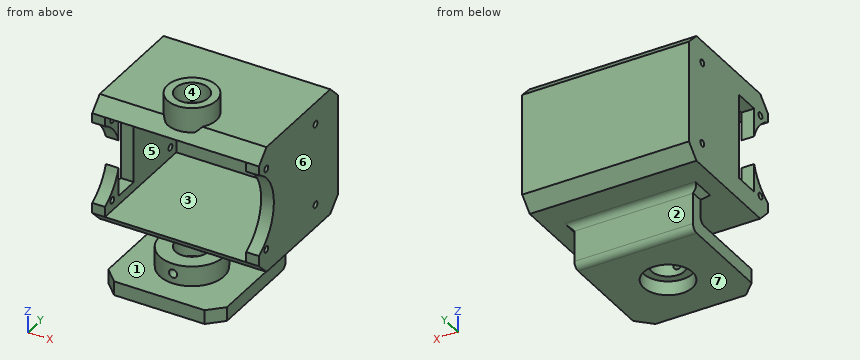
```python
from build123d import *

# Parameters (mm, degrees)
SKETCH1_W                       = 25
SKETCH1_H                       = 30
BOSS_EXTRUDE1_DEPTH             = 3.175
SKETCH2_W                       = 25
SKETCH2_H                       = 3.175
BOSS_EXTRUDE2_DEPTH             = 41.58
SKETCH3_W                       = 3.175
SKETCH3_H                       = 25
BOSS_EXTRUDE3_DEPTH             = 30
CUT_EXTRUDE1_REACH              = 60.775
SKETCH4_R                       = 11.5
CUT_EXTRUDE2_REACH              = 60.775
SKETCH5_R                       = 0.8
CUT_EXTRUDE3_REACH              = 60.775
SKETCH6_R                       = 0.8
SKETCH6_R_2                     = 0.799851166
SKETCH6_W                       = 21.2
SKETCH6_H                       = 6.375
CUT_EXTRUDE4_REACH              = 60.775
SKETCH7_R                       = 11.5
BOSS_EXTRUDE4_DEPTH             = 0.2
SKETCH9_W                       = 41.58
SKETCH9_H                       = 33.175
BOSS_EXTRUDE5_DEPTH             = 3.175
BOSS_EXTRUDE6_DEPTH             = 0.2
SKETCH11_W                      = 41.58
SKETCH11_H                      = 33.175
BOSS_EXTRUDE7_DEPTH             = 3.175
CHAMFER1_SIZE                   = 3.175
CHAMFER2_SIZE                   = 3.175
SKETCH13_W                      = 29.58
SKETCH13_H                      = 3.175
BOSS_EXTRUDE8_DEPTH             = 7.695
BOSS_EXTRUDE9_REACH             = 59.968
SKETCH14_W                      = 29.58
SKETCH14_H                      = 3.5
BOSS_EXTRUDE9_DIRECTION_2_DEPTH = 25
CHAMFER3_SIZE                   = 3.5
FILLET1_R                       = 1.5875
FILLET2_R                       = 1.5875
CUT_EXTRUDE5_REACH              = 70.161
SKETCH16_R                      = 6.1
SKETCH20_R                      = 8
SKETCH20_R_2                    = 4.1
BOSS_EXTRUDE11_DEPTH            = 5
CUT_EXTRUDE6_START              = -21.7275
SKETCH21_R                      = 1.025
CUT_EXTRUDE6_DEPTH              = 16
BOSS_EXTRUDE12_DEPTH            = 5
BOSS_EXTRUDE12_DEPTH_BACK       = 1.2
SKETCH23_R                      = 6.1
SKETCH23_R_2                    = 4.1
CHAMFER4_SIZE                   = 1.5


with BuildPart() as part:
    # Sketch1 → Boss-Extrude1 (new body)
    with BuildSketch(Plane(origin=(0, 0, 0), x_dir=(0, 0, -1), z_dir=(1, 0, 0))):
        with Locations((12.5, 15)):
            Rectangle(SKETCH1_W, SKETCH1_H)
    extrude(amount=BOSS_EXTRUDE1_DEPTH)

    # Sketch2 → Boss-Extrude2 (add)
    with BuildSketch(Plane.ZY):
        with Locations((-12.5, 31.5875)):
            Rectangle(SKETCH2_W, SKETCH2_H)
    extrude(amount=-BOSS_EXTRUDE2_DEPTH)

    # Sketch3 → Boss-Extrude3 (add)
    with BuildSketch(Plane.XZ.offset(-30)):
        with Locations((39.9925, -12.5)):
            Rectangle(SKETCH3_W, SKETCH3_H)
    extrude(amount=BOSS_EXTRUDE3_DEPTH)

    # Sketch4 → Cut-Extrude1 (cut, up to next)
    with BuildSketch(Plane.ZY, mode=Mode.PRIVATE) as cut_extrude1_sk1:
        with Locations((-12.359999929, -5.209996254)):
            Circle(SKETCH4_R)
    cut_extrude1_tool1 = extrude(cut_extrude1_sk1.sketch, amount=-CUT_EXTRUDE1_REACH, mode=Mode.PRIVATE) & part.part
    add(cut_extrude1_tool1.solids().sort_by_distance((0, -5.209996, -12.36))[0], mode=Mode.SUBTRACT)

    # Sketch5 → Cut-Extrude2 (cut, up to next)
    with BuildSketch(Plane.ZY, mode=Mode.PRIVATE) as cut_extrude2_sk1:
        with Locations((-22.609999929, 3.090003746)):
            Circle(SKETCH5_R)
    cut_extrude2_tool1 = extrude(cut_extrude2_sk1.sketch, amount=-CUT_EXTRUDE2_REACH, mode=Mode.PRIVATE) & part.part
    # Sketch5 → Cut-Extrude2 (cut, up to next)
    with BuildSketch(Plane.ZY, mode=Mode.PRIVATE) as cut_extrude2_sk2:
        with Locations((-22.609999929, 23.790003746)):
            Circle(SKETCH5_R)
    cut_extrude2_tool2 = extrude(cut_extrude2_sk2.sketch, amount=-CUT_EXTRUDE2_REACH, mode=Mode.PRIVATE) & part.part
    # Sketch5 → Cut-Extrude2 (cut, up to next)
    with BuildSketch(Plane.ZY, mode=Mode.PRIVATE) as cut_extrude2_sk3:
        with Locations((-2.109999929, 23.790003746)):
            Circle(SKETCH5_R)
    cut_extrude2_tool3 = extrude(cut_extrude2_sk3.sketch, amount=-CUT_EXTRUDE2_REACH, mode=Mode.PRIVATE) & part.part
    # Sketch5 → Cut-Extrude2 (cut, up to next)
    with BuildSketch(Plane.ZY, mode=Mode.PRIVATE) as cut_extrude2_sk4:
        with Locations((-2.109999929, 3.090003746)):
            Circle(SKETCH5_R)
    cut_extrude2_tool4 = extrude(cut_extrude2_sk4.sketch, amount=-CUT_EXTRUDE2_REACH, mode=Mode.PRIVATE) & part.part
    add(cut_extrude2_tool1.solids().sort_by_distance((0, 3.090004, -22.61))[0], mode=Mode.SUBTRACT)
    add(cut_extrude2_tool2.solids().sort_by_distance((0, 23.790004, -22.61))[0], mode=Mode.SUBTRACT)
    add(cut_extrude2_tool3.solids().sort_by_distance((0, 23.790004, -2.11))[0], mode=Mode.SUBTRACT)
    add(cut_extrude2_tool4.solids().sort_by_distance((0, 3.090004, -2.11))[0], mode=Mode.SUBTRACT)

    # Sketch6 → Cut-Extrude3 (cut, up to next)
    with BuildSketch(Plane(origin=(41.58, 0, 0), x_dir=(0, 0, -1), z_dir=(1, 0, 0)), mode=Mode.PRIVATE) as cut_extrude3_sk1:
        with Locations(Location((2.109999929, 3.090003746, 0), (0, 0, 180))):
            Circle(SKETCH6_R)
    cut_extrude3_tool1 = extrude(cut_extrude3_sk1.sketch, amount=-CUT_EXTRUDE3_REACH, mode=Mode.PRIVATE) & part.part
    # Sketch6 → Cut-Extrude3 (cut, up to next)
    with BuildSketch(Plane(origin=(41.58, 0, 0), x_dir=(0, 0, -1), z_dir=(1, 0, 0)), mode=Mode.PRIVATE) as cut_extrude3_sk2:
        with Locations(Location((22.609999929, 3.090003746, 0), (0, 0, 180))):
            Circle(SKETCH6_R)
    cut_extrude3_tool2 = extrude(cut_extrude3_sk2.sketch, amount=-CUT_EXTRUDE3_REACH, mode=Mode.PRIVATE) & part.part
    # Sketch6 → Cut-Extrude3 (cut, up to next)
    with BuildSketch(Plane(origin=(41.58, 0, 0), x_dir=(0, 0, -1), z_dir=(1, 0, 0)), mode=Mode.PRIVATE) as cut_extrude3_sk3:
        with Locations((22.609999929, 27.540003746)):
            Circle(SKETCH6_R_2)
    cut_extrude3_tool3 = extrude(cut_extrude3_sk3.sketch, amount=-CUT_EXTRUDE3_REACH, mode=Mode.PRIVATE) & part.part
    # Sketch6 → Cut-Extrude3 (cut, up to next)
    with BuildSketch(Plane(origin=(41.58, 0, 0), x_dir=(0, 0, -1), z_dir=(1, 0, 0)), mode=Mode.PRIVATE) as cut_extrude3_sk4:
        with Locations((2.109999929, 27.540003746)):
            Circle(SKETCH6_R)
    cut_extrude3_tool4 = extrude(cut_extrude3_sk4.sketch, amount=-CUT_EXTRUDE3_REACH, mode=Mode.PRIVATE) & part.part
    # Sketch6 → Cut-Extrude3 (cut, up to next)
    with BuildSketch(Plane(origin=(41.58, 0, 0), x_dir=(0, 0, -1), z_dir=(1, 0, 0)), mode=Mode.PRIVATE) as cut_extrude3_sk5:
        with Locations((12.359999929, 8.927503746)):
            Rectangle(SKETCH6_W, SKETCH6_H)
    cut_extrude3_tool5 = extrude(cut_extrude3_sk5.sketch, amount=-CUT_EXTRUDE3_REACH, mode=Mode.PRIVATE) & part.part
    add(cut_extrude3_tool1.solids().sort_by_distance((41.58, 3.090004, -2.11))[0], mode=Mode.SUBTRACT)
    add(cut_extrude3_tool2.solids().sort_by_distance((41.58, 3.090004, -22.61))[0], mode=Mode.SUBTRACT)
    add(cut_extrude3_tool3.solids().sort_by_distance((41.58, 27.540004, -22.61))[0], mode=Mode.SUBTRACT)
    add(cut_extrude3_tool4.solids().sort_by_distance((41.58, 27.540004, -2.11))[0], mode=Mode.SUBTRACT)
    add(cut_extrude3_tool5.solids().sort_by_distance((41.58, 8.927504, -12.36))[0], mode=Mode.SUBTRACT)

    # Sketch7 → Cut-Extrude4 (cut, up to next)
    with BuildSketch(Plane(origin=(41.58, 0, 0), x_dir=(0, 0, -1), z_dir=(1, 0, 0)), mode=Mode.PRIVATE) as cut_extrude4_sk1:
        with Locations((12.359999929, -5.209996254)):
            Circle(SKETCH7_R)
    cut_extrude4_tool1 = extrude(cut_extrude4_sk1.sketch, amount=-CUT_EXTRUDE4_REACH, mode=Mode.PRIVATE) & part.part
    add(cut_extrude4_tool1.solids().sort_by_distance((41.58, -5.209996, -12.36))[0], mode=Mode.SUBTRACT)

    # Sketch8 → Boss-Extrude4 (add)
    with BuildSketch(Plane.XY):
        Polygon((0, 33.175), (0, 0), (3.175, 0), (3.175, 30), (38.405, 30), (38.405, 0), (41.58, 0), (41.58, 33.175), align=None)
    extrude(amount=BOSS_EXTRUDE4_DEPTH)

    # Sketch9 → Boss-Extrude5 (add)
    with BuildSketch(Plane.XY.offset(0.2)):
        with Locations((20.79, 16.5875)):
            Rectangle(SKETCH9_W, SKETCH9_H)
    extrude(amount=BOSS_EXTRUDE5_DEPTH)

    # Sketch10 → Boss-Extrude6 (add)
    with BuildSketch(Plane(origin=(0, 0, -25), x_dir=(-1, 0, 0), z_dir=(0, 0, -1))):
        Polygon((0, 0), (0, 33.175), (-41.58, 33.175), (-41.58, 0), (-38.405, 0), (-38.405, 30), (-3.175, 30), (-3.175, 0), align=None)
    extrude(amount=BOSS_EXTRUDE6_DEPTH)

    # Sketch11 → Boss-Extrude7 (add)
    with BuildSketch(Plane(origin=(0, 0, -25.2), x_dir=(-1, 0, 0), z_dir=(0, 0, -1))):
        with Locations((-20.79, 16.5875)):
            Rectangle(SKETCH11_W, SKETCH11_H)
    extrude(amount=BOSS_EXTRUDE7_DEPTH)

    # Chamfer1
    chamfer1_edges = [part.edges().sort_by_distance(p)[0] for p in [
        (20.79, 33.175, 3.375),
        (20.79, 33.175, -28.375),
    ]]
    chamfer(chamfer1_edges, length=CHAMFER1_SIZE)

    # Chamfer2
    chamfer2_edges = [part.edges().sort_by_distance(p)[0] for p in [
        (20.79, 0, 3.375),
        (20.79, 0, -28.375),
    ]]
    chamfer(chamfer2_edges, length=CHAMFER2_SIZE - 0.0001)  # a hair under: the kernel refuses the full size

    # Sketch13 → Boss-Extrude8 (add)
    with BuildSketch(Plane(origin=(0, 0, -28.375), x_dir=(-1, 0, 0), z_dir=(0, 0, -1))):
        with Locations((-20.79, 19.7625)):
            Rectangle(SKETCH13_W, SKETCH13_H)
    extrude(amount=BOSS_EXTRUDE8_DEPTH)

    # Boss-Extrude9: up to this face of the body (flat: up to its plane)
    boss_extrude9_end = Plane(part.part.faces().sort_by_distance((20.79, 21.35, -32.2225))[0])
    # Sketch14 → Boss-Extrude9 (add, up to the picked face)
    with BuildSketch(Plane.XZ.offset(-18.175), mode=Mode.PRIVATE) as boss_extrude9_sk1:
        with Locations((20.79, -37.495)):
            Rectangle(SKETCH14_W, SKETCH14_H)
    boss_extrude9_tool1 = split(extrude(boss_extrude9_sk1.sketch, amount=-BOSS_EXTRUDE9_REACH, mode=Mode.PRIVATE), bisect_by=boss_extrude9_end, keep=Keep.BOTH, mode=Mode.PRIVATE)
    add(boss_extrude9_tool1.solids().sort_by(Axis((20.79, 18.175, -37.495), (0, 1, 0)))[0])

    # Sketch14 → Boss-Extrude9 direction 2 (add)
    with BuildSketch(Plane.XZ.offset(-18.175)):
        with Locations((20.79, -37.495)):
            Rectangle(SKETCH14_W, SKETCH14_H)
    extrude(amount=BOSS_EXTRUDE9_DIRECTION_2_DEPTH)

    # Chamfer3
    chamfer3_edges = [part.edges().sort_by_distance(p)[0] for p in [
        (6, -6.825, -37.495),
        (35.58, -6.825, -37.495),
    ]]
    chamfer(chamfer3_edges, length=CHAMFER3_SIZE)

    # Fillet1
    fillet1_edges = [part.edges().sort_by_distance(p)[0] for p in [
        (20.79, 18.175, -35.745),
        (20.79, 21.35, -39.245),
    ]]
    fillet(fillet1_edges, radius=FILLET1_R)

    # Fillet2
    fillet2_edges = [part.edges().sort_by_distance(p)[0] for p in [
        (20.79, 21.35, -28.375),
    ]]
    fillet(fillet2_edges, radius=FILLET2_R)

    # Sketch16 → Cut-Extrude5 (cut, up to next)
    with BuildSketch(Plane(origin=(0, 0, -39.245), x_dir=(-1, 0, 0), z_dir=(0, 0, -1)), mode=Mode.PRIVATE) as cut_extrude5_sk1:
        with Locations((-20.79, 6.9025)):
            Circle(SKETCH16_R)
    cut_extrude5_tool1 = extrude(cut_extrude5_sk1.sketch, amount=-CUT_EXTRUDE5_REACH, mode=Mode.PRIVATE) & part.part
    add(cut_extrude5_tool1.solids().sort_by_distance((20.79, 6.9025, -39.245))[0], mode=Mode.SUBTRACT)

    # Sketch20 → Boss-Extrude11 (add)
    with BuildSketch(Plane.XY.offset(-35.745)):
        with Locations(Location((20.79, 6.9025, 0), (0, 0, 180))):
            Circle(SKETCH20_R)
        with Locations((20.79, 6.9025)):
            Circle(SKETCH20_R_2, mode=Mode.SUBTRACT)
    extrude(amount=BOSS_EXTRUDE11_DEPTH)

    # Sketch21 → Cut-Extrude6 (cut)
    with BuildSketch(Plane.XZ.offset(6.825).offset(CUT_EXTRUDE6_START)):
        with Locations(Location((20.79, -33.245, 0), (0, 0, 270))):
            Circle(SKETCH21_R)
    extrude(amount=CUT_EXTRUDE6_DEPTH, mode=Mode.SUBTRACT)

    # Sketch23 → Boss-Extrude12 (add, two sides: drawn at the far end of the back side and taken through both)
    with BuildSketch(Plane.XY.offset(3.375).offset(-BOSS_EXTRUDE12_DEPTH_BACK)):
        with Locations(Location((20.79, 6.9025, 0), (0, 0, 180))):
            Circle(SKETCH23_R)
        with Locations((20.79, 6.9025)):
            Circle(SKETCH23_R_2, mode=Mode.SUBTRACT)
    extrude(amount=BOSS_EXTRUDE12_DEPTH + BOSS_EXTRUDE12_DEPTH_BACK)

    # Chamfer4
    chamfer4_edges = [part.edges().sort_by_distance(p)[0] for p in [
        (35.58, 20.55625, -28.375),
        (20.79, 18.175, -28.375),
        (6, 20.55625, -28.375),
    ]]
    chamfer(chamfer4_edges, length=CHAMFER4_SIZE)


with BuildPart() as body_2:
    # Mirror1: mirrored copy
    add(part.part.mirror(Plane(origin=(51.58, 0, 0), x_dir=(0, 0, 1), z_dir=(1, 0, 0))))


solid = body_2.part
```
The model under review builds one solid part; all positions refer to its coordinate system, in mm. Face numbers are marked on the shaded views. A direction names the side the tool comes from. Give positions to 0.01 mm unless a question says otherwise; leave off trailing zeros. Write each loop counter-clockwise with the first axis right and the second up, starting at its lowest first coordinate (ties: lowest second). Pieces come first, ordered by that corner, then holes. Notation, with made-up numbers: (2, -10) - (31, -10) arc R32 ccw to (31, 20) - close; hole circle Ø8 at (-8, 67.25). An arc over 180 degrees is marked (long way). Answer in a Markdown table with one row per item. Add a question column.
1. We need section D-D on z = -12. Write out the cut boundary in (x, y) (3 decimals), then the cut area to 3 significant figures.
2. We need section C-C on x = 82.37. State how many separate pieces and enclosed holes the cut face has, then the cut area to 3 significant figures.
3. We need section A-A on z = -20. Write out the cut boundary in (x, y) (3 decimals).
4. Tool access review of the marked faces 1, 2, 3 and 4: name each direction out of +Z, -Z, +X, -X, +Y, -Y from which nothing blocks a thin tool from reaching the whole face with its end or side.
5. Draft analysis for pull direction Z (two halves, no side actions). For the marked faces 5, 6 and 7, state which applies: +Z half, -Z half, draft (parallel to the pull), parting line (faces both ways), or undercut.
6. Insertion check: P1, Ø8, axis at x = 96.5, z = -9.5, coming from the -Y side; P2, Ø0.9, axis at x = 83.5, y = 1.5, coming from the -Z side (3 decimals); P3, Ø2.5, axis at y = 3.09, z = -22.61, coming from the +X side; P4, Ø10, axis at x = 67.5, y = 1, coming from the +Z side (3 decimals). Each pin has a flat end and moves straight along its axis. Give the tip position at first contact, or say it passes through.
7. Wall thickness on line 1 along Y through (x, z) = (101.65, -22.61) (3 decimals); line 2 along Z through (x, y) = (90.5, 5) (3 decimals); line 3 along Y through (x, z) = (63, -2) (3 decimals): over which ranges is each line inside the solid? List them lowest first. Write a range as [from, to].
Ans:
| question | item | result |
|---|---|---|
| 1 | outline | (61.58, 12.115) - (64.755, 12.115) - (64.755, 30) - (99.985, 30) - (99.985, 6.284) - (103.16, 6.284) - (103.16, 33.175) - (61.58, 33.175) - close |
| 1 | area | 264 mm^2 |
| 2 | separate pieces | 4 |
| 2 | enclosed holes | 0 |
| 2 | area | 397 mm^2 |
| 3 | outline | (61.58, 3.385) - (64.755, 3.385) - (64.755, 5.74) - (61.58, 5.74) - close; (61.58, 12.115) - (64.755, 12.115) - (64.755, 30) - (99.985, 30) - (99.985, 3.385) - (103.16, 3.385) - (103.16, 33.175) - (61.58, 33.175) - close |
| 4 | face 1 | none |
| 4 | face 2 | -Z, +X, -X, +Y |
| 4 | face 3 | -Y |
| 4 | face 4 | +Z |
| 5 | face 5 | undercut |
| 5 | face 6 | draft |
| 5 | face 7 | -Z half |
| 6 | P1 | stops at y = 5.23 |
| 6 | P2 | stops at z = -35.745 |
| 6 | P3 | stops at x = 103.16 |
| 6 | P4 | stops at z = 3.375 |
| 7 | line 1 | y = [0.004, 2.29], [3.89, 22.99], [24.59, 33.175] |
| 7 | line 2 | z = [-39.245, -35.745], [-28.375, -25.2], [0.2, 3.375] |
| 7 | line 3 | y = [0, 2.298], [3.882, 5.74], [12.115, 26.748], [28.332, 33.175] |
